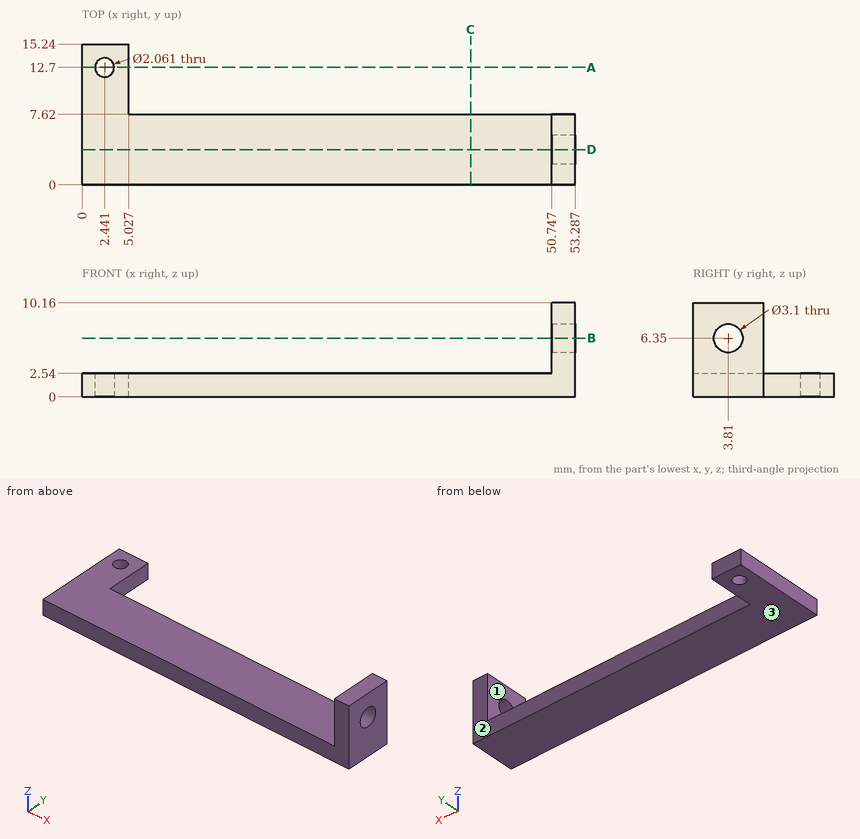
Drawing for the job (mm, zero at the part's lowest x, y, z). A direction names the side the tool comes from. Round coordinates to 2 decimals unless told otherwise and drop trailing zeros. Write each loop counter-clockwise with the first axis right and the second up, starting at its lowest first coordinate (ties: lowest second). Pieces come first, ordered by that corner, then holes. Notation, with made-up numbers: M 81,-4.75 L 89,-4.75 A26 ccw 89,34.25 Z; hole C 8.25,51 d1. An arc over 180 degrees is marked long. One line per question, with ' | ' between items.
1. Cut at D-D on y = 3.81. Write the cut outline in (x, z).
Working result:
outline: M 0,0 L 53.29,0 L 53.29,4.8 L 50.75,4.8 L 50.75,2.54 L 0,2.54 Z; M 50.75,7.9 L 53.29,7.9 L 53.29,10.16 L 50.75,10.16 Z
2. Cut at C-C on x = 42. Write the cut outline in (y, z).
Working result:
outline: M 0,0 L 7.62,0 L 7.62,2.54 L 0,2.54 Z
3. Cut at B-B on z = 6.35. Write the cut outline in (x, y).
Working result:
outline: M 50.75,0 L 53.29,0 L 53.29,2.26 L 50.75,2.26 Z; M 50.75,5.36 L 53.29,5.36 L 53.29,7.62 L 50.75,7.62 Z
4. Cut at A-A on y = 12.7. Write the cut outline in (x, z).
Working result:
outline: M 0,0 L 1.41,0 L 1.41,2.54 L 0,2.54 Z; M 3.47,0 L 5.03,0 L 5.03,2.54 L 3.47,2.54 Z
5. Which spindle directions (+Z, -Z, +X, -X, +Y, -Y) get a long thin tool onto all of the face, cutting with end or side? Do the marked faces 1, 2 and 3. Say none if no direction does.
Working result:
face 1: +Z, -X, +Y, -Y | face 2: +Z, -Z, +X, +Y | face 3: -Z, +X, -X, +Y, -Y
6. Probe L1, parallel to Y at x = 51.45, z = 6.35; L2, parallel to X at y = 3.5, z = 9.75; L3, parallel to Y at x = 6, z = 1.5. List the from-to ranges inside material, lowest first. Write a range as from..to.
Working result:
L1: 0..2.26, 5.36..7.62 | L2: 50.75..53.29 | L3: 0..7.62
7. Pin check, flat tips, straight feed: pin 1 Ø3 at (x, z) = (20.5, 5) entering from +Y; pin 2 Ø1 at (x, z) = (37, 1.5) entering from +Y; pin 3 Ø5 at (x, y) = (43, 9) entering from +Z; pin 4 Ø5 at (y, z) = (3.81, 6.35) entering from -X. Stop position of each tip, or through.
Working result:
pin 1: through | pin 2: y = 7.62 | pin 3: z = 2.54 | pin 4: x = 50.75
